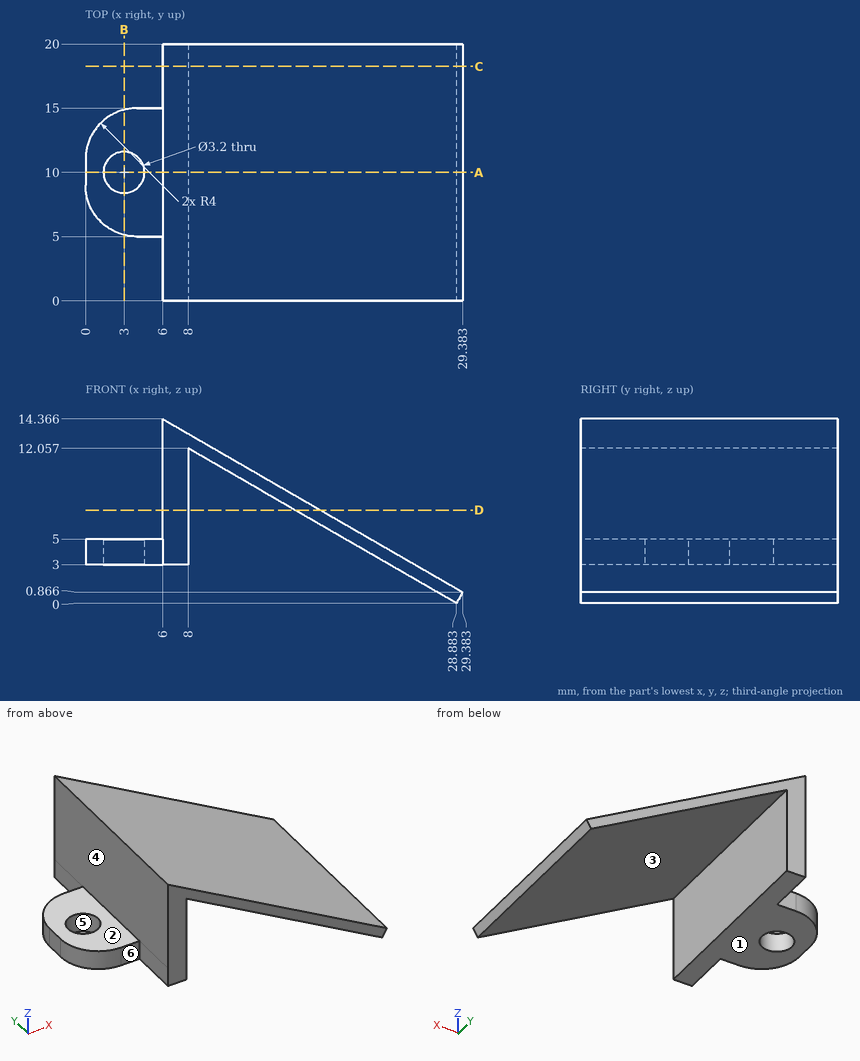
Answer from the drawing. Dimensions are ordinates in mm from the lowest x, y and z of the part. A direction names the side the tool comes from. Give positions to 0.01 mm unless a question says otherwise; leave off trailing zeros. Order: outer loops, then holes, each group sorted by start corner. A loop starts at its lowest first (then second) coordinate and runs counter-clockwise, first axis right, second up.
(1) Find section B-B (x = 3). Give the vertices of the cut face in (y, z), plus the area to 3 significant figures.
(2) For a pull along Y with two mould halves and no side action, classify the marked faces 4, 5 and 6 as released by +Y, released by -Y, zero draft, split by the parting line, or undercut.
(3) Find section C-C (y = 18.25). Give the vertices of the cut face in (x, z).
(4) Straight lines are drawn through the part: L1, parallel to X at y = 10, z = 3.45 (1 decimal); L2, parallel to X at y = 10, z = 4.45 (1 decimal); L3, parallel to Y at x = 3, z = 4.05. For each, find the intervals that lie inside material, in ascending order.
(5) Given pin 1 (0.6 mm diameter, centred on y = 3, z = 4, fed in from -X); pin 2 (4 mm diameter, centred on x = 3, y = 10, fed in from +Z); pin 3 (6 mm diameter, centred on y = 8.5, z = 3.5, fed in from +X), each flat-ended and moving along its own axis, determine where each tip first touches the part or whether it passes through.
(6) Find section D-D (z = 7.25). Give the vertices of the cut face in (x, y) (1 decimal).
(7) Find section A-A (y = 10). Give the vertices of the cut face in (x, z).
(8) For the marked faces 1, 2 and 3, determine the directions among +Z, -Z, +X, -X, +Y, -Y from which every point of the face is accessible in a straight line to the end or side of a thin tool.
Result sheet:
1. outline: (5.13, 3) - (8.4, 3) - (8.4, 5) - (5.13, 5) - close; (11.6, 3) - (14.87, 3) - (14.87, 5) - (11.6, 5) - close
1. area: 13.1 mm2
2. face 4: zero draft
2. face 5: undercut
2. face 6: released by -Y
3. outline: (6, 3) - (8, 3) - (8, 12.06) - (28.88, 0) - (29.38, 0.87) - (6, 14.37) - close
4. L1: x = 0 to 1.4, 4.6 to 8, 22.9 to 24.9
4. L2: x = 0 to 1.4, 4.6 to 8, 21.2 to 23.2
4. L3: y = 5.13 to 8.4, 11.6 to 14.87
5. pin 1: stops at x = 6
5. pin 2: stops at z = 5
5. pin 3: stops at x = 29.38
6. outline: (6, 0) - (8, 0) - (8, 20) - (6, 20) - close; (16.3, 0) - (18.3, 0) - (18.3, 20) - (16.3, 20) - close
7. outline: (0, 3) - (1.4, 3) - (1.4, 5) - (0, 5) - close; (4.6, 3) - (8, 3) - (8, 12.06) - (28.88, 0) - (29.38, 0.87) - (6, 14.37) - (6, 5) - (4.6, 5) - close
8. face 1: -Z, -X, +Y, -Y
8. face 2: +Z, -X, +Y, -Y
8. face 3: -Z, +Y, -Y
